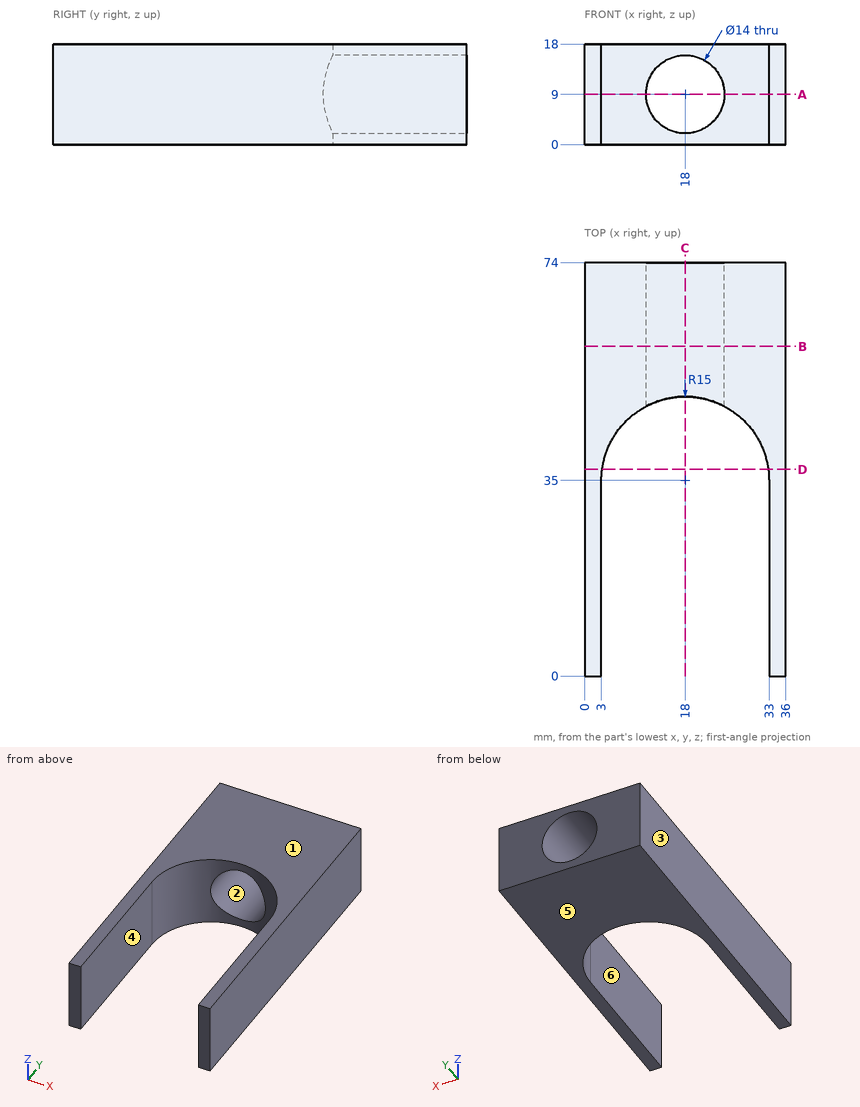
Geometry check sheet. Reference: drawing and pictorial views, mm from the part's lowest x, y, z. A direction names the side the tool comes from. Round coordinates to 2 decimals unless told otherwise and drop trailing zeros. Order: outer loops, then holes, each group sorted by start corner. A loop starts at its lowest first (then second) coordinate and runs counter-clockwise, first axis right, second up. Notation, with made-up numbers: (16, 15) - (62, 15) arc R12 ccw to (62, 34) - close; hole circle Ø11 at (16.25, -40). An arc over 180 degrees is marked (long way). Use a Markdown table: item, result. Add a question column.
1) Section check C-C (x = 18). Record the cut outline in (y, z).
2) Section check D-D (y = 37). Record the cut outline in (x, z).
3) Set-up check for the marked faces 5 and 6: record each of +Z, -Z, +X, -X, +Y, -Y from which the full face is reachable in a straight line by a thin tool's end or side.
4) Section check B-B (y = 59). Record the cut outline in (x, z), then the cut area to 3 significant figures.
5) Gauge pin test, flat end, axial feed: P1, Ø5, axis at x = 25, z = 12.5, coming from the -Y side. Record the tip position at first contact, or that the pin passes through.
6) Thickness scan on line 1 along Z through (x, y) = (18, 62.75); line 2 along X through (y, z) = (57.5, 9); line 3 along X through (y, z) = (14, 11). Record the ranges inside material, lowest first.
7) Section check A-A (z = 9). Record the cut outline in (x, y), then the cut area to 3 significant figures.
8) Mould release check, pull along X, two halves, no side actions. Record for the marked faces 1, 2, 3 and 4: released by +X, released by -X, zero draft, split by the parting line, or undercut.
Established:
| question | item | result |
|---|---|---|
| 1 | outline | (50, 0) - (74, 0) - (74, 2) - (50, 2) - close; (50, 16) - (74, 16) - (74, 18) - (50, 18) - close |
| 2 | outline | (0, 0) - (3.13, 0) - (3.13, 18) - (0, 18) - close; (32.87, 0) - (36, 0) - (36, 18) - (32.87, 18) - close |
| 3 | face 5 | -Z, +X, -X, +Y, -Y |
| 3 | face 6 | +Z, -Z, -Y |
| 4 | outline | (0, 0) - (36, 0) - (36, 18) - (0, 18) - close; hole circle Ø14 at (18, 9) |
| 4 | area | 494 mm2 |
| 5 | P1 | y = 46.61 |
| 6 | line 1 | 0 to 2, 16 to 18 |
| 6 | line 2 | 0 to 11, 25 to 36 |
| 6 | line 3 | 0 to 3, 33 to 36 |
| 7 | outline | (0, 0) - (3, 0) - (3, 35) arc R15 cw to (11, 48.27) - (11, 74) - (0, 74) - close; (25, 48.27) arc R15 cw to (33, 35) - (33, 0) - (36, 0) - (36, 74) - (25, 74) - close |
| 7 | area | 917 mm2 |
| 8 | face 1 | zero draft |
| 8 | face 2 | undercut |
| 8 | face 3 | released by -X |
| 8 | face 4 | undercut |
